Design review of the part built by this model. Coordinates are the model's own, in mm. A direction names the side the tool comes from. Round coordinates to 2 decimals unless told otherwise and drop trailing zeros. Loops run counter-clockwise (first coordinate to the right, second up) from the corner with the lowest first, then second, coordinate; pieces in that order, holes last. Notation, with made-up numbers: (44, -9.5) - (96, -9.5) arc R19 ccw to (96, 14.5) - close; hole circle Ø8 at (50.25, 67). An arc over 180 degrees is marked (long way). Answer as CSV lines item,"result". Start each with the question number.
(1) Wall thickness on L1, parallel to Z at x = 48, y = -1.5; L2, parallel to X at y = 0.25, z = -24; L3, parallel to X at y = 5.5, z = -27.5: over which ranges is each line inside the solid? List them lowest first.
(2) Consider section C-C (x = 31). Give the boundary of the cut face in (y, z).
(3) Mouldability with a two-part tool opening along Z and no side actions: class faces 3 (the cylindrical face through (56.58, 0.09, -32.39)), 4 (the flat face through (-25, 8, -1)), 5 (the cylindrical face through (-43.83, -0.47, 27.19)) as released by +Z, released by -Z, zero draft, split by the parting line, or undercut.
(4) For faces 1 (the cylindrical face through (52.17, -0.47, -20.81)), 2 (the flat face through (42, 6.5, -1)), list the 3-axis set-ups (+Z, -Z, +X, -X, +Y, -Y) from which the entire face can be reached by the end or side of a thin tool; tool diameter is ignored.
(5) Consider section A-A (y = 0.5). Give the boundary of the cut face in (x, z).
(6) Consider section B-B (z = 0.5). Give the boundary of the cut face in (x, y).
(7) Consider section D-D (z = -28). Count the separate pieces of the cut face and the enclosed holes in it, and give its area (3 significant figures).
(8) For P1, Ø17.5, axis at x = 48, z = 15.5, coming from the +Y side; P2, Ø1.5, axis at y = 8.5, z = -4.5, coming from the -X side; P3, Ø0.9, axis at y = 8.5, z = -11.5, coming from the +X side; P4, Ø2, axis at y = 6.5, z = -24.5, coming from the -X side, all flat-tipped, find the tip position at first contact; note any pin that passes through.
from build123d import *

# Parameters (mm, degrees)
BOSS_EXTRUDE1_DEPTH              = 36
BOSS_EXTRUDE1_DEPTH_BACK         = 36
SKETCH1_W                        = 120
SKETCH1_H                        = 13
SKETCH1_W_2                      = 50
SKETCH1_H_2                      = 3
FILLET1_R                        = 12
M12X1_5_TAPPED_HOLE1_D           = 10.5
M12X1_5_TAPPED_HOLE1_CSINK_D     = 12.05
M12X1_5_TAPPED_HOLE1_CSINK_ANGLE = 90


with BuildPart() as part:
    # Sketch1 → Boss-Extrude1 (new, two sides: drawn at the far end of the back side and taken through both)
    with BuildSketch(Plane.XY.offset(-BOSS_EXTRUDE1_DEPTH_BACK)):
        Rectangle(SKETCH1_W, SKETCH1_H)
        with Locations((0, 8)):
            Rectangle(SKETCH1_W_2, SKETCH1_H_2)
    extrude(amount=BOSS_EXTRUDE1_DEPTH + BOSS_EXTRUDE1_DEPTH_BACK)

    # Fillet1
    fillet1_edges = [part.edges().sort_by_distance(p)[0] for p in [
        (60, 0, 36),
        (-60, 0, 36),
        (60, 0, -36),
        (-60, 0, -36),
    ]]
    fillet(fillet1_edges, radius=FILLET1_R)

    # M12x1.5 Tapped Hole1 (through all)
    with Locations(Plane(origin=(0, 6.5, 0), x_dir=(1, 0, 0), z_dir=(0, 1, 0))):
        with Locations((-48, -24), (-48, 24), (48, 24), (48, -24)):
            CounterSinkHole(M12X1_5_TAPPED_HOLE1_D / 2, M12X1_5_TAPPED_HOLE1_CSINK_D / 2, counter_sink_angle=M12X1_5_TAPPED_HOLE1_CSINK_ANGLE)


solid = part.part
Determined:
1,L1,"z = -36 to -29.25, -18.75 to 18.75, 29.25 to 36"
1,L2,"x = -60 to -53.25, -42.75 to 42.75, 53.25 to 60"
1,L3,"x = -59.48 to -51.91, -44.09 to 44.09, 51.91 to 59.48"
2,outline,"(-6.5, -36) - (6.5, -36) - (6.5, 36) - (-6.5, 36) - close"
3,face 3,"released by -Z"
3,face 4,"zero draft"
3,face 5,"undercut"
4,face 1,"+Y, -Y"
4,face 2,"+Z, -Z, +X, +Y"
5,outline,"(-60, -24) arc R12 ccw to (-48, -36) - (48, -36) arc R12 ccw to (60, -24) - (60, 24) arc R12 ccw to (48, 36) - (-48, 36) arc R12 ccw to (-60, 24) - close; hole circle Ø10.5 at (-48, -24); hole circle Ø10.5 at (-48, 24); hole circle Ø10.5 at (48, -24); hole circle Ø10.5 at (48, 24)"
6,outline,"(-60, -6.5) - (60, -6.5) - (60, 6.5) - (25, 6.5) - (25, 9.5) - (-25, 9.5) - (-25, 6.5) - (-60, 6.5) - close"
7,separate pieces,"3"
7,enclosed holes,"0"
7,area,"1,510 mm^2"
8,P1,"stops at y = 6.5"
8,P2,"stops at x = -25"
8,P3,"stops at x = 25"
8,P4,"stops at x = -60"
